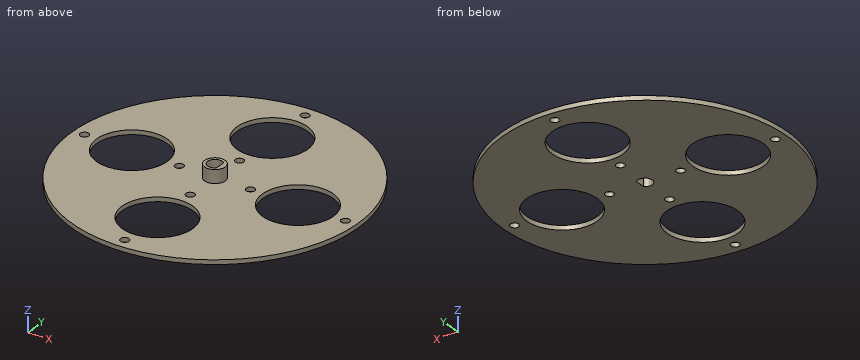
Autodesk Fusion 360 part; units mm, degrees
sketch "Sketch1" plane through (0, 0, 0) normal (0, 0, 1) x (1, 0, 0)
  circle A0 centre (0, 0) radius 2.5
  circle A1 centre (0, 0) radius 1.775
  circle A2 centre (0, 0) radius 3.5
  line L0 (1.775, 0) -> (1.775, 3.0165)
  line L1 (1.775, 0) -> (1.775, -3.0165)
  circle A3 centre (0, 0) radius 48.5
  circle A4 centre (0, 44.6993) radius 1.45
  circle A5 centre (0, 44.6993) radius 1.45
  circle A6 centre (0, 12.1993) radius 1.45
  circle A7 centre (0, 28.4493) radius 12
  circle A8 centre (-44.6993, 0) radius 1.45
  circle A9 centre (-28.4493, 0) radius 12
  circle A10 centre (-12.1993, 0) radius 1.45
  circle A11 centre (0, -44.6993) radius 1.45
  circle A12 centre (0, -28.4493) radius 12
  circle A13 centre (0, -12.1993) radius 1.45
  circle A14 centre (44.6993, 0) radius 1.45
  circle A15 centre (28.4493, 0) radius 12
  circle A16 centre (12.1993, 0) radius 1.45
  point P0 (0, 47.6993)
  point P1 (0, 28.4493)
  dimension "d1" = 5
  dimension "d3" = 3.55
  dimension "d4" = 7
  dimension "d5" = 97
  dimension "d7" = 2.9
  dimension "d8" = 32.5
  dimension "d9" = 2.9
  dimension "d10" = 2.9
  dimension "d11" = 24
  dimension "d13" = 360
extrude "Extrude4" add sketch "Sketch1" along normal blind 6 contours A0 L0 L1 | A0 A2 L0 L1 | A0 A2 L0 L1 picked at (2.2513, 0.1082) makes body 1
extrude "Extrude3" add sketch "Sketch1" along normal blind 2 separate body contours A0 L0 L1 | A0 A2 L0 L1 | A0 A2 L0 L1 picked at (2.2513, 0.1082) makes body 2
extrude "Extrude5" add sketch "Sketch1" along normal blind 1.5 contours A3 bodies 1 2
Verification items for the finished model (mm, model axes). Coordinates: 2 decimals unless noted, no trailing zeros. Write each loop counter-clockwise with the first axis right and the second up, starting at its lowest first coordinate (ties: lowest second). Pieces come first, ordered by that corner, then holes. Notation, with made-up numbers: (46.5, 38.5) - (77.5, 38.5) arc R31 ccw to (77.5, 65.5) - close; hole circle Ø5 at (-11.5, 88). An arc over 180 degrees is marked (long way). Answer as a JSON object with one key per item and string values.
(1) Cross-section at B-B on y = -38.5. Record the cut outline in (x, z).
Report:
{"outline": "(-29.5, 0) - (-6.56, 0) - (-6.56, 1.5) - (-29.5, 1.5) - close; (6.56, 0) - (29.5, 0) - (29.5, 1.5) - (6.56, 1.5) - close"}
(2) Thickness scan on line 1 along Y through (x, z) = (-4.5, 1) (3 decimals); line 2 along Z through (x, y) = (26, -24); line 3 along X through (y, z) = (-3.5, 1.1). Record the ranges inside material, lowest first.
Report:
{"line 1": "-48.291 to -39.574, -17.325 to 17.325, 39.574 to 48.291", "line 2": "0 to 1.5", "line 3": "-48.37 to -39.93, -16.97 to 16.97, 39.93 to 48.37"}
(3) Cross-section at D-D on x = 0. Give the number of separate pieces and of enclosed holes in the cut face, plus the area to 3 significant figures.
Report:
{"separate pieces": "8", "enclosed holes": "0", "area": "57.6 mm^2"}
(4) Cross-section at A-A on x = -21.5. Record the cut outline in (y, z), plus the area to 3 significant figures.
Report:
{"outline": "(-43.47, 0) - (-9.78, 0) - (-9.78, 1.5) - (-43.47, 1.5) - close; (9.78, 0) - (43.47, 0) - (43.47, 1.5) - (9.78, 1.5) - close", "area": "101 mm^2"}
(5) Gauge pin test, flat ends, axial feed: pin 1 Ø2 at (x, z) = (23, 3) entering from -Y; pin 2 Ø1.1 at (y, z) = (0.5, 3.5) entering from -X; pin 3 Ø1.5 at (x, z) = (-30, 0.5) entering from +Y; pin 4 Ø4.5 at (x, y) = (0, 44.7) entering from +Z. Record the tip position at first contact, or that the pin passes through.
Report:
{"pin 1": "through", "pin 2": "x = -3.5", "pin 3": "y = 38.69", "pin 4": "z = 1.5"}
(6) Cross-section at C-C on z = 4.15. Record the cut outline in (x, y) (1 decimal).
Report:
{"outline": "circle Ø7 at (0, 0); hole (1.8, -1.8) - (1.8, 1.8) arc R2.5 ccw (long way) to start"}
